Autodesk Inventor part; units mm, degrees
ref_plane "YZ Plane" through (0, 0, 0) normal (1, 0, 0) x (0, 1, 0)
ref_plane "XZ Plane" through (0, 0, 0) normal (0, 1, 0) x (-1, 0, 0)
ref_plane "XY Plane" through (0, 0, 0) normal (0, 0, 1) x (1, 0, 0)
sketch "Эскиз1" plane through (0, 0, 0) normal (0, 0, 1) x (1, 0, 0)
  circle A0 centre (0, 0) radius 55
  dimension "d0" = 110
extrude "Выдавливание1" add sketch "Эскиз1" along normal blind 230
sketch "Эскиз2" plane through (0, 0, 0) normal (0, 1, 0) x (-1, 0, 0)
  line L0 (55, 0) -> (-55, 0)
  line L1 (-55, 0) -> (-55, 230)
  line L2 (55, 230) -> (-55, 230)
  line L3 (-55, 230) -> (-55, 222.5)
  line L4 (-55, 222.5) -> (-52, 222.5)
  line L5 (-52, 222.5) -> (-52, 226)
  line L6 (-52, 226) -> (-55, 226)
  line L7 (0, -46) -> (0, 276)
  line L8 (-55, 0) -> (-55, 7.5)
  line L9 (-55, 0) -> (-55, 230)
  line L10 (-55, 7.5) -> (-52, 7.5)
  line L11 (-52, 7.5) -> (-52, 4)
  line L12 (-52, 4) -> (-55, 4)
  line L13 (-55, 0) -> (-55, 230)
  line L14 (-55, 7.5) -> (-55, 27.5)
  line L15 (-55, 0) -> (-55, 230)
  line L16 (-55, 27.5) -> (-53, 27.5)
  line L17 (-53, 27.5) -> (-53, 33.5)
  line L18 (-53, 33.5) -> (-55, 33.5)
  line L19 (-55, 0) -> (-55, 230)
  line L20 (-55, 222.5) -> (-55, 202.5)
  line L21 (-55, 0) -> (-55, 230)
  line L22 (-55, 202.5) -> (-53, 202.5)
  line L23 (-53, 202.5) -> (-53, 196.5)
  line L24 (-53, 196.5) -> (-55, 196.5)
  line L25 (-55, 0) -> (-55, 230)
  line L26 (-55, 0) -> (-55, 230)
  line L27 (-55, 55) -> (-55, 106)
  line L28 (-55, 0) -> (-55, 230)
  line L29 (-55, 106) -> (-53, 106)
  line L30 (-53, 106) -> (-53, 124)
  line L31 (-53, 124) -> (-55, 124)
  line L32 (-55, 0) -> (-55, 230)
  point P0 (0, 0)
  dimension "d3" = 7.5
  dimension "d5" = 7.5
  dimension "d6" = 3.5
  dimension "d7" = 20
  dimension "d8" = 2
  dimension "d9" = 6
  dimension "d10" = 20
  dimension "d11" = 2
  dimension "d12" = 6
  dimension "d13" = 51
  dimension "d14" = 18
revolve "Вращение1" cut sketch "Эскиз2" angle 360 about axis through (0, 0, -10) along (0, 0, 1) contours L1 L10 L11 L12 | L6 L5 L4 L1 | L1 L18 L17 L16 | L22 L23 L24 L1 | L1 L31 L30 L29
sketch "Эскиз3" plane through (0, 0, 0) normal (1, 0, 0) x (0, 1, 0)
  line L0 (-53, 27.5) -> (-53, 33.5)
  line L1 (-53, 33.5) -> (53, 33.5)
  line L2 (55, 33.5) -> (-55, 33.5)
  line L3 (0, 33.5) -> (0, 30.5)
  circle A0 centre (0, 30.5) radius 1
  line L4 (-53, 106) -> (53, 106)
  line L5 (0, 106) -> (0, 115)
  circle A1 centre (0, 115) radius 1
  line L6 (-53, 196.5) -> (53, 196.5)
  line L7 (0, 196.5) -> (0, 199.5)
  circle A2 centre (0, 199.5) radius 1
  point P0 (0, 0)
  dimension "d15" = 2
  dimension "d16" = 3
extrude "Выдавливание2" cut sketch "Эскиз3" against normal through all both and the other way through all
sketch "Эскиз4" plane through (0, 0, 0) normal (0, 1, 0) x (-1, 0, 0)
  line L0 (-53, 29.5) -> (53, 29.5)
  line L1 (0, 29.5) -> (0, 30.5)
  circle A0 centre (0, 30.5) radius 1
  line L2 (-53, 114) -> (53, 114)
  line L3 (0, 114) -> (0, 115)
  circle A1 centre (0, 115) radius 1
  line L4 (-53, 198.5) -> (53, 198.5)
  line L5 (0, 198.5) -> (0, 199.5)
  circle A2 centre (0, 199.5) radius 1
  point P0 (0, 0)
  dimension "d19" = 1
  dimension "d20" = 1
extrude "Выдавливание3" cut sketch "Эскиз4" against normal through all both and the other way through all
properties part number "Палец" material "Сталь, высокопрочная, низколегированная"
Input: part model. Units: mm. Frame: model coordinates. A direction names the side the tool comes from. Coordinates: 2 decimals unless noted, no trailing zeros. Loops run counter-clockwise (first coordinate to the right, second up) from the corner with the lowest first, then second, coordinate; pieces in that order, holes last.
Q1. Section A-A, the plane z = 158.5. Return the cut outline in (x, y), and give its area (3 significant figures).
Results are:
outline: circle Ø110 at (0, 0)
area: 9,500 mm2
Q2. Section B-B, the plane x = -21.5. Give the number of separate pieces and of enclosed holes in the cut face, and give its area (3 significant figures).
Results are:
separate pieces: 1
enclosed holes: 3
area: 23,100 mm2
Q3. Contact query for flat-ended pins moving along their axis: pin 1 (8 mm diameter, centred on x = -33, z = 60, fed in from +Y); pin 2 (10 mm diameter, centred on x = 37.5, z = 98, fed in from -Y); pin 3 (2 mm diameter, centred on x = 29, z = 35.5, fed in from -Y). Output: stop coordinate, or through.
Results are:
pin 1: stops at y = 46.73
pin 2: stops at y = -44.37
pin 3: stops at y = -47.34
Q4. Line query: line 1 along Z through (x, y) = (23, 0); line 2 along Z through (x, y) = (-29, 46); line 3 along Y through (x, z) = (1, 160.5). Output: solid intervals per line, ascending.
Results are:
line 1: z = 0 to 29.5, 31.5 to 114, 116 to 198.5, 200.5 to 230
line 2: z = 0 to 4, 7.5 to 27.5, 33.5 to 106, 124 to 196.5, 202.5 to 222.5, 226 to 230
line 3: y = -54.99 to 54.99
Q5. Set-up query: faces 1 (the cylindrical face through (-11.923, 53.692, 212.36)), 2 (the flat face through (-29, 45, 202.5)). Return all of +Z, -Z, +X, -X, +Y, -Y with unobstructed straight access to the full face (end or side cutting, diameter ignored); none if empty.
Results are:
face 1: +Z, -Z
face 2: none
Q6. Mould query, pull axis Z, two halves, no side actions, for faces 3 (the flat face through (-1, 1, 230)), 4 (the cylindrical face through (-11.923, 53.692, 1.972)), 5 (the cylindrical face through (-41.265, 31.641, 5.726)). Classes: +Z half, -Z half, draft (parallel to the pull), parting line (faces both ways), or undercut.
Results are:
face 3: +Z half
face 4: draft
face 5: undercut
